Check sheet for the modelled part. Datum: model origin and axes. Units: mm. Coordinates: 2 decimals unless noted, no trailing zeros. Loops run counter-clockwise (first coordinate to the right, second up) from the corner with the lowest first, then second, coordinate; pieces in that order, holes last.
```python
from build123d import *

# Parameters (mm, degrees)
SKETCH1_W           = 311.15
SKETCH1_H           = 80.191313252
BOSS_EXTRUDE1_DEPTH = 1


with BuildPart() as part:
    # Sketch1 → Boss-Extrude1 (new body)
    with BuildSketch(Plane(origin=(0, 0, 0), x_dir=(1, 0, 0), z_dir=(0, 1, 0))):
        with Locations((155.575, 40.095656626)):
            Rectangle(SKETCH1_W, SKETCH1_H)
        Polygon((12.7, 52.8066), (18.310796472, 52.8066), (27.609157985, 67.491313252), (12.7, 67.491313252), align=None, mode=Mode.SUBTRACT)
        Polygon((12.7, 12.7), (27.609157985, 12.7), (18.310796472, 27.384713252), (12.7, 27.384713252), align=None, mode=Mode.SUBTRACT)
        Polygon((39.78500573, 12.7), (112.61499427, 12.7), (127.635, 37.424696429), (127.635, 42.599313252), (112.61499427, 67.491313252), (39.78500573, 67.491313252), (24.765, 42.599313252), (24.765, 37.424696429), align=None, mode=Mode.SUBTRACT)
        Polygon((134.089203528, 27.384713252), (139.081919808, 27.384713252), (148.242867112, 12.7), (124.790842015, 12.7), align=None, mode=Mode.SUBTRACT)
        Polygon((124.790842015, 67.491313252), (134.089203528, 52.8066), (139.081919808, 52.8066), (148.242867112, 67.491313252), align=None, mode=Mode.SUBTRACT)
        Polygon((160.625882169, 67.376840045), (242.726117831, 67.376840045), (257.937, 42.599313252), (257.937, 37.424696429), (242.987396137, 12.586149763), (160.364603863, 12.586149763), (145.415, 37.424696429), (145.415, 42.599313252), align=None, mode=Mode.SUBTRACT)
        Polygon((255.109132888, 67.491313252), (264.270080192, 52.8066), (269.262796472, 52.8066), (278.561157985, 67.491313252), align=None, mode=Mode.SUBTRACT)
        Polygon((264.270080192, 27.384713252), (269.262796472, 27.384713252), (278.561157985, 12.7), (255.109132888, 12.7), align=None, mode=Mode.SUBTRACT)
        Polygon((298.45, 67.491313252), (298.45, 12.7), (290.73700573, 12.7), (275.717, 37.424696429), (275.717, 42.599313252), (290.73700573, 67.491313252), align=None, mode=Mode.SUBTRACT)
    extrude(amount=BOSS_EXTRUDE1_DEPTH)


solid = part.part
```
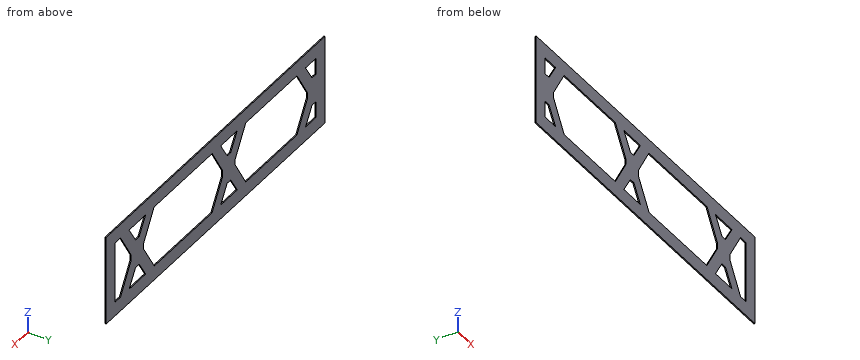
1) Section check D-D on x = 193. Enter the section's corners in (y, z).
Answer sheet:
outline: (0, -80.19) - (1, -80.19) - (1, -67.38) - (0, -67.38) - close; (0, -12.59) - (1, -12.59) - (1, 0) - (0, 0) - close
2) Section check C-C on z = -49.5. Enter the section's corners in (x, y), plus the area to 3 significant figures.
Answer sheet:
outline: (0, 0) - (28.93, 0) - (28.93, 1) - (0, 1) - close; (123.47, 0) - (149.65, 0) - (149.65, 1) - (123.47, 1) - close; (253.7, 0) - (279.88, 0) - (279.88, 1) - (253.7, 1) - close; (298.45, 0) - (311.15, 0) - (311.15, 1) - (298.45, 1) - close
area: 94.0 mm2
3) Scan lines: line 1 (X direction, y = 0.5, z = -38.5) (3 decimals); line 2 (Z direction, x = 177, y = 0.8); line 3 (Z direction, x = 70, y = 0.3). Record each from-to range of solid material in increasing order.
Answer sheet:
line 1: x = 0 to 24.765, 127.635 to 145.415, 257.937 to 275.717, 298.45 to 311.15
line 2: z = -80.19 to -67.38, -12.59 to 0
line 3: z = -80.19 to -67.49, -12.7 to 0
4) Section check B-B on z = -18. Enter the section's corners in (x, y), plus the area to 3 significant figures.
Answer sheet:
outline: (0, 0) - (12.7, 0) - (12.7, 1) - (0, 1) - close; (24.25, 0) - (36.57, 0) - (36.57, 1) - (24.25, 1) - close; (115.83, 0) - (128.15, 0) - (128.15, 1) - (115.83, 1) - close; (144.94, 0) - (157.11, 0) - (157.11, 1) - (144.94, 1) - close; (246.25, 0) - (258.42, 0) - (258.42, 1) - (246.25, 1) - close; (275.21, 0) - (287.52, 0) - (287.52, 1) - (275.21, 1) - close; (298.45, 0) - (311.15, 0) - (311.15, 1) - (298.45, 1) - close
area: 86.7 mm2
5) Depth check by flat-ended pin: pin 1 (6 mm diameter, centred on x = 74, z = -69, fed in from -Y). Enter the tip coordinate at first touch or a pass-through.
Answer sheet:
pin 1: stops at y = 0
6) Section check A-A on x = 59.5. Enter the section's corners in (y, z).
Answer sheet:
outline: (0, -80.19) - (1, -80.19) - (1, -67.49) - (0, -67.49) - close; (0, -12.7) - (1, -12.7) - (1, 0) - (0, 0) - close
